Geometry check sheet. Reference: the model listing, model coordinates, mm. A direction names the side the tool comes from. Coordinates: 2 decimals unless noted, no trailing zeros. Loops run counter-clockwise (first coordinate to the right, second up) from the corner with the lowest first, then second, coordinate; pieces in that order, holes last. Notation, with made-up numbers: (-25.75, -4) - (25.25, -4) arc R23 ccw to (25.25, 14) - close; hole circle Ø5 at (27.25, 0.25). An arc over 180 degrees is marked (long way). Write item = value, one per line. Start each with the question number.
from build123d import *

# Parameters (mm, degrees)
SKETCH1_W           = 150
SKETCH1_H           = 30
BOSS_EXTRUDE1_DEPTH = 7
SKETCH2_R           = 8.492301233
SKETCH2_R_2         = 8.746428368
SKETCH2_R_3         = 7.993391254
SKETCH2_W           = 146.177010272
SKETCH2_H           = 1.023518213
BOSS_EXTRUDE2_DEPTH = 1
SKETCH3_W           = 10.614560987
SKETCH3_H           = 22.545060987
SKETCH3_W_2         = 4.652355514
SKETCH3_W_3         = 4.001025742
SKETCH3_W_4         = 3.814931522
SKETCH3_W_5         = 4.466261294
SKETCH3_W_6         = 4.652355515
BOSS_EXTRUDE3_DEPTH = 20
SKETCH4_W           = 44.01124784
SKETCH4_H           = 10.469759529
BOSS_EXTRUDE4_DEPTH = 55
SKETCH5_R           = 2.698367098
BOSS_EXTRUDE5_DEPTH = 15


with BuildPart() as part:
    # Sketch1 → Boss-Extrude1 (new body)
    with BuildSketch(Plane(origin=(0, 0, 0), x_dir=(1, 0, 0), z_dir=(0, 1, 0))):
        with Locations((75, 15)):
            Rectangle(SKETCH1_W, SKETCH1_H)
    extrude(amount=BOSS_EXTRUDE1_DEPTH)

    # Sketch2 → Boss-Extrude2 (add)
    with BuildSketch(Plane(origin=(0, 7, 0), x_dir=(1, 0, 0), z_dir=(0, 1, 0))):
        with Locations(Location((46.015825143, 16.53527732, 0), (0, 0, 90))):
            Circle(SKETCH2_R)
        with Locations(Location((79.69887907, 16.53527732, 0), (0, 0, 90))):
            Circle(SKETCH2_R_2)
        with Locations(Location((110.497472577, 16.53527732, 0), (0, 0, 90))):
            Circle(SKETCH2_R_3)
        with Locations((75.372188441, 5.974430301)):
            Rectangle(SKETCH2_W, SKETCH2_H)
    extrude(amount=BOSS_EXTRUDE2_DEPTH)

    # Sketch3 → Boss-Extrude3 (add)
    with BuildSketch(Plane.XZ):
        with Locations((144.692719506, -18.727469507)):
            Rectangle(SKETCH3_W, SKETCH3_H)
        with Locations((134.131438592, -18.727469507)):
            Rectangle(SKETCH3_W_2, SKETCH3_H)
        with Locations((125.617628, -18.727469507)):
            Rectangle(SKETCH3_W_3, SKETCH3_H)
        with Locations((117.801670735, -18.727469507)):
            Rectangle(SKETCH3_W_4, SKETCH3_H)
        with Locations((109.939189915, -18.727469507)):
            Rectangle(SKETCH3_W_5, SKETCH3_H)
        with Locations((101.844091319, -18.727469507)):
            Rectangle(SKETCH3_W_6, SKETCH3_H)
        with Locations((48.155908681, -18.727469507)):
            Rectangle(SKETCH3_W_6, SKETCH3_H)
        with Locations((40.060810085, -18.727469507)):
            Rectangle(SKETCH3_W_5, SKETCH3_H)
        with Locations((32.198329265, -18.727469507)):
            Rectangle(SKETCH3_W_4, SKETCH3_H)
        with Locations((24.382372, -18.727469507)):
            Rectangle(SKETCH3_W_3, SKETCH3_H)
        with Locations((15.868561408, -18.727469507)):
            Rectangle(SKETCH3_W_2, SKETCH3_H)
        with Locations((5.307280494, -18.727469507)):
            Rectangle(SKETCH3_W, SKETCH3_H)
    extrude(amount=BOSS_EXTRUDE3_DEPTH)

    # Sketch4 → Boss-Extrude4 (add)
    with BuildSketch(Plane.XZ):
        with Locations((75, -21.677122954)):
            Rectangle(SKETCH4_W, SKETCH4_H)
    extrude(amount=BOSS_EXTRUDE4_DEPTH)

    # Sketch5 → Boss-Extrude5 (add)
    with BuildSketch(Plane.XZ.offset(55)):
        with Locations(Location((74.767407147, -21.559835962, 0), (0, 0, 270))):
            Circle(SKETCH5_R)
    extrude(amount=BOSS_EXTRUDE5_DEPTH)


solid = part.part
(1) Sectioned sample at A-A on y = -8.5. Count the separate pieces of the cut face and the enclosed holes in it, plus the area to 3 significant figures.
(2) Scan lines: line 1 (X direction, y = -30.5, z = -18); line 2 (Y direction, x = 35, z = -17); line 3 (Y direction, x = 118, z = -27.5). Record each from-to range of solid material in increasing order.
(3) Sectioned sample at D-D on y = -40.5. Enter the section's corners in (x, z).
(4) Tool access check on faces 4 (the face through (134, -20, -19)), 5 (the face through (30.291, -10, -19)), 6 (the face through (85.021, 7.493, -9.594)), 7 (the face through (126, -10, -7.455)). Record the directions out of +Z, -Z, +X, -X, +Y, -Y that give a thin tool (end or side, any length) a straight path to the whole face; none if there is none.
(5) Sectioned sample at C-C on z = -2.5. Enter the section's corners in (x, y), plus the area to 3 significant figures.
(6) Depth check by flat-ended pin: pin 1 (4 mm diameter, centred on y = -57.5, z = -20, fed in from +X); pin 2 (3 mm diameter, centred on x = 117, z = -22.5, fed in from -Y); pin 3 (1.3 mm diameter, centred on x = 41, y = -8, fed in from +Z). Enter the tip coordinate at first touch or a pass-through.
(7) Draft check along X on faces 1 (the face through (13.542, -10, -19)), 2 (the face through (0, -7, -18)), 3 (the face through (32, -20, -19)). Enter one of: pulls with the +X half, pulls with the -X half, needs draft (parallel to the pull), parting line crosses it, or undercut.
(8) Sectioned sample at B-B on x = 56.5. Enter the section's corners in (y, z).
Working result:
q1.separate_pieces = 13
q1.enclosed_holes = 0
q1.area = 1,910 mm2
q2.line_1 = 52.99 to 97.01
q2.line_2 = 0 to 7
q2.line_3 = -20 to 7
q3.outline = (52.99, -26.91) - (97.01, -26.91) - (97.01, -16.44) - (52.99, -16.44) - close
q4.face_4 = +Z, -Z, +X, -Y
q4.face_5 = +Z, -Z, -Y
q4.face_6 = +Y
q4.face_7 = +Z, +X, -X, -Y
q5.outline = (0, 0) - (150, 0) - (150, 7) - (0, 7) - close
q5.area = 1,050 mm2
q6.pin_1 = 77.47
q6.pin_2 = -20
q6.pin_3 = -7.45
q7.face_1 = undercut
q7.face_2 = pulls with the -X half
q7.face_3 = needs draft
q8.outline = (-55, -26.91) - (0, -26.91) - (0, -30) - (7, -30) - (7, -6.49) - (8, -6.49) - (8, -5.46) - (7, -5.46) - (7, 0) - (0, 0) - (0, -16.44) - (-55, -16.44) - close
